```python
from build123d import *
from OCP.BRepFilletAPI import BRepFilletAPI_MakeChamfer

# Parameters (mm, degrees)
SKETCH_1_W          = 55
SKETCH_1_H          = 25
EXTRUDE_1_DEPTH     = 10
SKETCH_2_W          = 20.4
SKETCH_2_H          = 1.4
CUT_EXTRUDE_1_DEPTH = 2
SKETCH_3_W          = 7.5
SKETCH_3_H          = 9
CUT_EXTRUDE_2_DEPTH = 39.487010796
SKETCH_4_W          = 7.5
SKETCH_4_H          = 9
CUT_EXTRUDE_3_DEPTH = 39.487010796
CUT_EXTRUDE_4_DEPTH = 32.819805153
CUT_EXTRUDE_5_DEPTH = 32.819805153
SKETCH_7_W          = 20.995896459
SKETCH_7_H          = 1
EXTRUDE_2_DEPTH     = 0.8
SKETCH_8_W          = 20
SKETCH_8_H          = 1.5
CUT_EXTRUDE_6_DEPTH = 10
CHAMFER_1_SIZE      = 8
CHAMFER_1_SIZE2     = 7.5


with BuildPart() as part:
    # 草图1 → 凸台-拉伸1 (new body)
    with BuildSketch(Plane.XY):
        Rectangle(SKETCH_1_W, SKETCH_1_H)
    extrude(amount=-EXTRUDE_1_DEPTH)

    # 草图2 → 切除-拉伸1 (cut)
    with BuildSketch(Plane.XZ.offset(12.5)):
        with Locations((0, -2.5)):
            Rectangle(SKETCH_2_W, SKETCH_2_H)
    extrude(amount=-CUT_EXTRUDE_1_DEPTH, mode=Mode.SUBTRACT)

    # 草图3 → 切除-拉伸2 (cut, through all)
    with BuildSketch(Plane.XZ.offset(12.5)):
        with Locations((-23.75, -4.5)):
            Rectangle(SKETCH_3_W, SKETCH_3_H)
    extrude(amount=-CUT_EXTRUDE_2_DEPTH, mode=Mode.SUBTRACT)

    # 草图4 → 切除-拉伸3 (cut, through all)
    with BuildSketch(Plane.XZ.offset(12.5)):
        with Locations((23.75, -4.5)):
            Rectangle(SKETCH_4_W, SKETCH_4_H)
    extrude(amount=-CUT_EXTRUDE_3_DEPTH, mode=Mode.SUBTRACT)

    # 草图5 → 切除-拉伸4 (cut, through all)
    with BuildSketch(Plane(origin=(0, 0, -10), x_dir=(-1, 0, 0), z_dir=(0, 0, -1))):
        with BuildLine():
            Line((21.5, 1), (21.5, -5))
            ThreePointArc((21.5, -5), (23, -6.5), (24.5, -5))
            Line((24.5, -5), (24.5, 1))
            ThreePointArc((24.5, 1), (23, 2.5), (21.5, 1))
        make_face()
    extrude(amount=-CUT_EXTRUDE_4_DEPTH, mode=Mode.SUBTRACT)

    # 草图6 → 切除-拉伸5 (cut, through all)
    with BuildSketch(Plane(origin=(0, 0, -10), x_dir=(-1, 0, 0), z_dir=(0, 0, -1))):
        with BuildLine():
            Line((-24.5, 1), (-24.5, -5))
            ThreePointArc((-24.5, -5), (-23, -6.5), (-21.5, -5))
            Line((-21.5, -5), (-21.5, 1))
            ThreePointArc((-21.5, 1), (-23, 2.5), (-24.5, 1))
        make_face()
    extrude(amount=-CUT_EXTRUDE_5_DEPTH, mode=Mode.SUBTRACT)

    # 草图7 → 凸台-拉伸2 (add)
    with BuildSketch(Plane(origin=(0, 0, -2.8), x_dir=(-1, 0, 0), z_dir=(0, 0, -1))):
        with Locations((0.49794823, -13)):
            Rectangle(SKETCH_7_W, SKETCH_7_H)
    extrude(amount=-EXTRUDE_2_DEPTH)

    # 草图8 → 切除-拉伸6 (cut)
    with BuildSketch(Plane.XZ.offset(12.5)):
        with Locations((0, -8.25)):
            Rectangle(SKETCH_8_W, SKETCH_8_H)
    extrude(amount=-CUT_EXTRUDE_6_DEPTH, mode=Mode.SUBTRACT)

    # 倒角1: one chamfer whose edges measure the first distance from different faces: ONE call of the kernel's chamfer builder (chamfer() names one face for all edges)
    chamfer_1_edges_1 = [part.edges().sort_by_distance(p)[0] for p in [
        (27.5, 12.5, -9.5),
    ]]
    chamfer_1_side_1 = [part.faces().sort_by_distance(p)[0] for p in [
        (0, 12.5, -5.162650602),
    ]]
    chamfer_1_edges_2 = [part.edges().sort_by_distance(p)[0] for p in [
        (-27.5, 12.5, -9.5),
    ]]
    chamfer_1_side_2 = [part.faces().sort_by_distance(p)[0] for p in [
        (-27.5, 0, -9.5),
    ]]
    chamfer_1 = BRepFilletAPI_MakeChamfer(part.part.solid().wrapped)
    for e in chamfer_1_edges_1:
        chamfer_1.Add(CHAMFER_1_SIZE, CHAMFER_1_SIZE2, e.wrapped, chamfer_1_side_1[0].wrapped)  # the first distance lies on this face
    for e in chamfer_1_edges_2:
        chamfer_1.Add(CHAMFER_1_SIZE, CHAMFER_1_SIZE2, e.wrapped, chamfer_1_side_2[0].wrapped)  # the first distance lies on this face
    add(Compound.cast(chamfer_1.Shape()), mode=Mode.REPLACE)


solid = part.part
```
Verification items for the finished model (mm, model axes). A direction names the side the tool comes from. Give positions to 0.01 mm unless a question says otherwise; leave off trailing zeros. Order: outer loops, then holes, each group sorted by start corner. A loop starts at its lowest first (then second) coordinate and runs counter-clockwise, first axis right, second up. Notation, with made-up numbers: M 14.25,40 L 47.25,40 A22 cw 47.25,60 Z; hole C 41,32.25 d10. An arc over 180 degrees is marked long. Return JSON: item names as keys, results as strings. Group by question number.
1) Section check A-A on y = -3.75. Record the cut outline in (x, z).
2) Section check D-D on z = -5. Record the cut outline in (x, y).
3) Section check C-C on y = -9.25. Record the cut outline in (x, z).
4) Section check B-B on x = -23. Record the cut outline in (y, z), and give its area (3 significant figures).
5) Go/stop test with flat-tipped pins: pin 1 Ø5 at (y, z) = (2.5, -4) entering from -X; pin 2 Ø2.5 at (y, z) = (5.5, -4) entering from +X; pin 3 Ø3 at (x, z) = (13.5, -3.5) entering from -Y. Record where each tip stops, or that it passes through.
6) Mould release check, pull along Z, two halves, no side actions. Record for faces 5 (the face through (-23, -6.5, -9.5)), 6 (the face through (0, 0, -10)), 7 (the face through (0, -8, -7.5)), 8 (the face through (-25, -3, -9)): pulls with the +Z half, pulls with the -Z half, needs draft (parallel to the pull), parting line crosses it, or undercut.
7) Scan lines: line 1 (Z direction, x = -4.5, y = -4); line 2 (X direction, y = -5.5, z = -8.5); line 3 (X direction, y = 0.75, z = -8). Record each from-to range of solid material in increasing order.
8) Access from +Z, -Z, +X, -X, +Y, -Y to the whole of each face (thin tool, end or side, straight path). Record for faces 1 (the face through (0, -12, -3.2)), 2 (the face through (-10.2, -12, -3)), 3 (the face through (25, -3, -9)), 4 (the face through (0, -13, -2)).
Answer block:
{
 "1": {"outline": "M -27.5,-10 L -24.5,-10 L -24.5,-9 L -27.5,-9 Z; M -21.5,-10 L 21.5,-10 L 21.5,-9 L 20,-9 L 20,0 L -20,0 L -20,-9 L -21.5,-9 Z; M 24.5,-10 L 27.5,-10 L 27.5,-9 L 24.5,-9 Z; hole M -10,-9 L 10,-9 L 10,-7.5 L -10,-7.5 Z"},
 "2": {"outline": "M -20,-12.5 L 20,-12.5 L 20,12.03 L 19.5,12.5 L -20,12.5 Z"},
 "3": {"outline": "M -27.5,-10 L 27.5,-10 L 27.5,-9 L 20,-9 L 20,0 L -20,0 L -20,-9 L -27.5,-9 Z; hole M -10,-9 L 10,-9 L 10,-7.5 L -10,-7.5 Z"},
 "4": {"outline": "M -12.5,-10 L -6.5,-10 L -6.5,-9 L -12.5,-9 Z; M 2.5,-10 L 9.3,-10 L 9.3,-9 L 2.5,-9 Z", "area": "12.8 mm^2"},
 "5": {"pin 1": "stops at x = -20", "pin 2": "stops at x = 20", "pin 3": "stops at y = -12.5"},
 "6": {"face 5": "needs draft", "face 6": "pulls with the -Z half", "face 7": "undercut", "face 8": "pulls with the +Z half"},
 "7": {"line 1": "z = -10 to -9, -7.5 to 0", "line 2": "x = -20 to -10, 10 to 20", "line 3": "x = -20 to 20"},
 "8": {"face 1": "-Y", "face 2": "none", "face 3": "+Z, +X, +Y, -Y", "face 4": "+Z, +X, -X, -Y"}
}
